```python
from build123d import *

# Parameters (mm, degrees)
F1_DEPTH = 7
F2_R     = 3


with BuildPart() as f1:
    # F0 (on Top) → F1 (new body)
    with BuildSketch(Plane.XY):
        with BuildLine():
            ThreePointArc((11.139936974, 0.4736076595), (11.1474839596, 0.2368572775), (11.15, 0))
            ThreePointArc((11.15, 0), (11.1474839596, -0.2368572775), (11.139936974, -0.4736076595))
            ThreePointArc((11.139936974, -0.4736076595), (11.4562515521, -1.9356574125), (12.0547261732, -3.306595967))
            ThreePointArc((12.0547261732, -3.306595967), (12.3881814074, -1.6682210338), (12.5, 0))
            ThreePointArc((12.5, 0), (12.3881814074, 1.6682210338), (12.0547261732, 3.306595967))
            ThreePointArc((12.0547261732, 3.306595967), (11.4562515521, 1.9356574125), (11.139936974, 0.4736076595))
        make_face()
        with BuildLine():
            ThreePointArc((5.9801247516, 9.4106645863), (9.6561832522, 5.575), (11.139936974, 0.4736076595))
            ThreePointArc((11.139936974, 0.4736076595), (11.4562515521, 1.9356574125), (12.0547261732, 3.306595967))
            ThreePointArc((12.0547261732, 3.306595967), (10.8253175473, 6.25), (8.8909591941, 8.7864011181))
            ThreePointArc((8.8909591941, 8.7864011181), (7.4044542683, 8.9535761701), (5.9801247516, 9.4106645863))
        make_face()
        with BuildLine():
            ThreePointArc((12.0547261732, -3.306595967), (11.4562515521, -1.9356574125), (11.139936974, -0.4736076595))
            ThreePointArc((11.139936974, -0.4736076595), (9.6561832522, -5.575), (5.9801247516, -9.4106645863))
            ThreePointArc((5.9801247516, -9.4106645863), (7.4044542683, -8.9535761701), (8.8909591941, -8.7864011181))
            ThreePointArc((8.8909591941, -8.7864011181), (10.8253175473, -6.25), (12.0547261732, -3.306595967))
        make_face()
        with BuildLine():
            ThreePointArc((5.1598122224, 9.8842722458), (5.575, 9.6561832522), (5.9801247516, 9.4106645863))
            ThreePointArc((5.9801247516, 9.4106645863), (7.4044542683, 8.9535761701), (8.8909591941, 8.7864011181))
            ThreePointArc((8.8909591941, 8.7864011181), (6.25, 10.8253175473), (3.1637669791, 12.0929970852))
            ThreePointArc((3.1637669791, 12.0929970852), (4.0517972839, 10.8892335825), (5.1598122224, 9.8842722458))
        make_face()
        with BuildLine():
            ThreePointArc((8.8909591941, 8.7864011181), (10.8253175473, 6.25), (12.0547261732, 3.306595967))
            ThreePointArc((12.0547261732, 3.306595967), (13.8777539277, 5.4728270333), (16.3707526215, 6.8148198569))
            Line((16.3707526215, 6.8148198569), (17.8056945141, 4.3294275931))
            Line((17.8056945141, 4.3294275931), (26.4132363375, 15.2496891096))
            Line((26.4132363375, 15.2496891096), (12.6522415365, 13.2554699846))
            Line((12.6522415365, 13.2554699846), (14.087183429, 10.7700777209))
            ThreePointArc((14.087183429, 10.7700777209), (11.6784842052, 9.2820739322), (8.8909591941, 8.7864011181))
        make_face()
        with BuildLine():
            ThreePointArc((8.8909591941, -8.7864011181), (7.4044542683, -8.9535761701), (5.9801247516, -9.4106645863))
            ThreePointArc((5.9801247516, -9.4106645863), (5.575, -9.6561832522), (5.1598122224, -9.8842722458))
            ThreePointArc((5.1598122224, -9.8842722458), (4.0517972839, -10.8892335825), (3.1637669791, -12.0929970852))
            ThreePointArc((3.1637669791, -12.0929970852), (6.25, -10.8253175473), (8.8909591941, -8.7864011181))
        make_face()
        with BuildLine():
            ThreePointArc((16.3707526215, -6.8148198569), (13.8777539277, -5.4728270333), (12.0547261732, -3.306595967))
            ThreePointArc((12.0547261732, -3.306595967), (10.8253175473, -6.25), (8.8909591941, -8.7864011181))
            ThreePointArc((8.8909591941, -8.7864011181), (11.6784842052, -9.2820739322), (14.087183429, -10.7700777209))
            Line((14.087183429, -10.7700777209), (12.6522415365, -13.2554699846))
            Line((12.6522415365, -13.2554699846), (26.4132363375, -15.2496891096))
            Line((26.4132363375, -15.2496891096), (17.8056945141, -4.3294275931))
            Line((17.8056945141, -4.3294275931), (16.3707526215, -6.8148198569))
        make_face()
        with BuildLine():
            ThreePointArc((-5.1598122224, 9.8842722458), (0, 11.15), (5.1598122224, 9.8842722458))
            ThreePointArc((5.1598122224, 9.8842722458), (4.0517972839, 10.8892335825), (3.1637669791, 12.0929970852))
            ThreePointArc((3.1637669791, 12.0929970852), (0, 12.5), (-3.1637669791, 12.0929970852))
            ThreePointArc((-3.1637669791, 12.0929970852), (-4.0517972839, 10.8892335825), (-5.1598122224, 9.8842722458))
        make_face()
        with BuildLine():
            ThreePointArc((3.1637669791, -12.0929970852), (4.0517972839, -10.8892335825), (5.1598122224, -9.8842722458))
            ThreePointArc((5.1598122224, -9.8842722458), (0, -11.15), (-5.1598122224, -9.8842722458))
            ThreePointArc((-5.1598122224, -9.8842722458), (-4.0517972839, -10.8892335825), (-3.1637669791, -12.0929970852))
            ThreePointArc((-3.1637669791, -12.0929970852), (0, -12.5), (3.1637669791, -12.0929970852))
        make_face()
        with BuildLine():
            ThreePointArc((-5.9801247516, 9.4106645863), (-5.575, 9.6561832522), (-5.1598122224, 9.8842722458))
            ThreePointArc((-5.1598122224, 9.8842722458), (-4.0517972839, 10.8892335825), (-3.1637669791, 12.0929970852))
            ThreePointArc((-3.1637669791, 12.0929970852), (-6.25, 10.8253175473), (-8.8909591941, 8.7864011181))
            ThreePointArc((-8.8909591941, 8.7864011181), (-7.4044542683, 8.9535761701), (-5.9801247516, 9.4106645863))
        make_face()
        with BuildLine():
            ThreePointArc((-3.1637669791, 12.0929970852), (0, 12.5), (3.1637669791, 12.0929970852))
            ThreePointArc((3.1637669791, 12.0929970852), (2.1992697225, 14.7549009655), (2.2835691925, 17.5848975778))
            Line((2.2835691925, 17.5848975778), (5.1534529775, 17.5848975778))
            Line((5.1534529775, 17.5848975778), (0, 30.4993782192))
            Line((0, 30.4993782192), (-5.1534529775, 17.5848975778))
            Line((-5.1534529775, 17.5848975778), (-2.2835691925, 17.5848975778))
            ThreePointArc((-2.2835691925, 17.5848975778), (-2.1992697225, 14.7549009655), (-3.1637669791, 12.0929970852))
        make_face()
        with BuildLine():
            ThreePointArc((-3.1637669791, -12.0929970852), (-4.0517972839, -10.8892335825), (-5.1598122224, -9.8842722458))
            ThreePointArc((-5.1598122224, -9.8842722458), (-5.575, -9.6561832522), (-5.9801247516, -9.4106645863))
            ThreePointArc((-5.9801247516, -9.4106645863), (-7.4044542683, -8.9535761701), (-8.8909591941, -8.7864011181))
            ThreePointArc((-8.8909591941, -8.7864011181), (-6.25, -10.8253175473), (-3.1637669791, -12.0929970852))
        make_face()
        with BuildLine():
            ThreePointArc((2.2835691925, -17.5848975778), (2.1992697225, -14.7549009655), (3.1637669791, -12.0929970852))
            ThreePointArc((3.1637669791, -12.0929970852), (0, -12.5), (-3.1637669791, -12.0929970852))
            ThreePointArc((-3.1637669791, -12.0929970852), (-2.1992697225, -14.7549009655), (-2.2835691925, -17.5848975778))
            Line((-2.2835691925, -17.5848975778), (-5.1534529775, -17.5848975778))
            Line((-5.1534529775, -17.5848975778), (0, -30.4993782192))
            Line((0, -30.4993782192), (5.1534529775, -17.5848975778))
            Line((5.1534529775, -17.5848975778), (2.2835691925, -17.5848975778))
        make_face()
        with BuildLine():
            ThreePointArc((-11.139936974, 0.4736076595), (-9.6561832522, 5.575), (-5.9801247516, 9.4106645863))
            ThreePointArc((-5.9801247516, 9.4106645863), (-7.4044542683, 8.9535761701), (-8.8909591941, 8.7864011181))
            ThreePointArc((-8.8909591941, 8.7864011181), (-10.8253175473, 6.25), (-12.0547261732, 3.306595967))
            ThreePointArc((-12.0547261732, 3.306595967), (-11.4562515521, 1.9356574125), (-11.139936974, 0.4736076595))
        make_face()
        with BuildLine():
            ThreePointArc((-8.8909591941, -8.7864011181), (-7.4044542683, -8.9535761701), (-5.9801247516, -9.4106645863))
            ThreePointArc((-5.9801247516, -9.4106645863), (-9.6561832522, -5.575), (-11.139936974, -0.4736076595))
            ThreePointArc((-11.139936974, -0.4736076595), (-11.4562515521, -1.9356574125), (-12.0547261732, -3.306595967))
            ThreePointArc((-12.0547261732, -3.306595967), (-10.8253175473, -6.25), (-8.8909591941, -8.7864011181))
        make_face()
        with BuildLine():
            ThreePointArc((-11.139936974, -0.4736076595), (-11.15, 0), (-11.139936974, 0.4736076595))
            ThreePointArc((-11.139936974, 0.4736076595), (-11.4562515521, 1.9356574125), (-12.0547261732, 3.306595967))
            ThreePointArc((-12.0547261732, 3.306595967), (-12.5, 0), (-12.0547261732, -3.306595967))
            ThreePointArc((-12.0547261732, -3.306595967), (-11.4562515521, -1.9356574125), (-11.139936974, -0.4736076595))
        make_face()
        with BuildLine():
            ThreePointArc((-12.0547261732, 3.306595967), (-10.8253175473, 6.25), (-8.8909591941, 8.7864011181))
            ThreePointArc((-8.8909591941, 8.7864011181), (-11.6784842052, 9.2820739322), (-14.087183429, 10.7700777209))
            Line((-14.087183429, 10.7700777209), (-12.6522415365, 13.2554699846))
            Line((-12.6522415365, 13.2554699846), (-26.4132363375, 15.2496891096))
            Line((-26.4132363375, 15.2496891096), (-17.8056945141, 4.3294275931))
            Line((-17.8056945141, 4.3294275931), (-16.3707526215, 6.8148198569))
            ThreePointArc((-16.3707526215, 6.8148198569), (-13.8777539277, 5.4728270333), (-12.0547261732, 3.306595967))
        make_face()
        with BuildLine():
            ThreePointArc((-14.087183429, -10.7700777209), (-11.6784842052, -9.2820739322), (-8.8909591941, -8.7864011181))
            ThreePointArc((-8.8909591941, -8.7864011181), (-10.8253175473, -6.25), (-12.0547261732, -3.306595967))
            ThreePointArc((-12.0547261732, -3.306595967), (-13.8777539277, -5.4728270333), (-16.3707526215, -6.8148198569))
            Line((-16.3707526215, -6.8148198569), (-17.8056945141, -4.3294275931))
            Line((-17.8056945141, -4.3294275931), (-26.4132363375, -15.2496891096))
            Line((-26.4132363375, -15.2496891096), (-12.6522415365, -13.2554699846))
            Line((-12.6522415365, -13.2554699846), (-14.087183429, -10.7700777209))
        make_face()
    extrude(amount=F1_DEPTH)

    # F2
    f2_edges = [f1.edges().sort_by_distance(p)[0] for p in [
        (-19.532739, -14.25258, 0),
        (-22.109465, -9.789558, 0),
        (-22.109465, 9.789558, 0),
        (-19.532739, 14.25258, 0),
        (-2.576726, 24.042138, 0),
        (19.532739, 14.25258, 0),
        (22.109465, 9.789558, 0),
        (22.109465, -9.789558, 0),
        (19.532739, -14.25258, 0),
        (-2.576726, -24.042138, 0),
        (2.576726, -24.042138, 0),
        (2.576726, 24.042138, 0),
        (-19.532739, 14.25258, 7),
        (-22.109465, 9.789558, 7),
        (-2.576726, 24.042138, 7),
        (2.576726, 24.042138, 7),
        (22.109465, 9.789558, 7),
        (22.109465, -9.789558, 7),
        (19.532739, -14.25258, 7),
        (2.576726, -24.042138, 7),
        (-2.576726, -24.042138, 7),
        (-22.109465, -9.789558, 7),
        (-19.532739, -14.25258, 7),
        (19.532739, 14.25258, 7),
    ]]
    fillet(f2_edges, radius=F2_R)


solid = f1.part
```
Geometry check sheet. Reference: the model listing, model coordinates, mm. A direction names the side the tool comes from. Coordinates: 2 decimals unless noted, no trailing zeros. Order: outer loops, then holes, each group sorted by start corner. A loop starts at its lowest first (then second) coordinate and runs counter-clockwise, first axis right, second up.
Q1. Tool access check on faces 4 (the face through (20.802, 8.977, 1.306)), 5 (the face through (-3, 17.585, 3)), 6 (the face through (16.9, 5.9, 3.5)), 7 (the face through (-19.512, -13.72, 1.306)), 8 (the face through (3, 17.585, 3)). Record the directions out of +Z, -Z, +X, -X, +Y, -Y that give a thin tool (end or side, any length) a straight path to the whole face; none if there is none.
Reply:
face 4: -Z, +X
face 5: +Z, -Z, -X
face 6: +Z, -Z
face 7: -Z, -Y
face 8: +Z, -Z, +X
Q2. Sectioned sample at A-A on x = 8. Record the cut outline in (y, z), and give its area (3 significant figures).
Reply:
outline: (-9.6, 0) - (-7.77, 0) - (-7.77, 7) - (-9.6, 7) - close; (7.77, 0) - (9.6, 0) - (9.6, 7) - (7.77, 7) - close
area: 25.7 mm2
Q3. Draft check along Y on faces 1 (the face through (2.63, 22.5, 1.31)), 2 (the face through (-19.629, -14.267, 3.493)), 3 (the face through (-20.802, -8.977, 5.694)). Enter one of: released by +Y, released by -Y, zero draft, split by the parting line, or undercut.
Reply:
face 1: released by +Y
face 2: released by -Y
face 3: undercut
Q4. Sectioned sample at C-C on y = -16. Record the cut outline in (x, z), and give its area (3 significant figures).
Reply:
outline: (-2.1, 0) - (2.1, 0) - (2.1, 7) - (-2.1, 7) - close
area: 29.5 mm2
Q5. Thickness scan on probe 1 along Y at (x, z) = (13, 2.5); probe 2 along Y at (x, z) = (-8, 2.25); probe 3 along X at (y, z) = (8.5, 2.25). Record the ranges inside material, lowest first.
Reply:
probe 1: y = -13.26 to -12.65, -9.94 to -4.63, 4.63 to 9.94, 12.65 to 13.26
probe 2: y = -9.6 to -7.77, 7.77 to 9.6
probe 3: x = -20.97 to -7.22, 7.22 to 20.97
Q6. Sectioned sample at B-B on y = 2.5. Record the cut outline in (x, z).
Reply:
outline: (-12.25, 0) - (-10.87, 0) - (-10.87, 7) - (-12.25, 7) - close; (10.87, 0) - (12.25, 0) - (12.25, 7) - (10.87, 7) - close
Q7. Depth check by flat-ended pin: pin 1 Ø4 at (y, z) = (4.5, 3.5) entering from -X; pin 2 Ø2 at (x, z) = (13.5, 3.5) entering from -Y; pin 3 Ø1.5 at (x, y) = (12.5, -13) entering from +Z. Enter the tip coordinate at first touch or a pass-through.
Reply:
pin 1: stops at x = -19.52
pin 2: stops at y = -13.52
pin 3: stops at z = 6.03
